CAD build for the part. Positions are in the model's coordinates, mm. A direction names the side the tool comes from. Coordinates: 2 decimals unless noted, no trailing zeros. Loops run counter-clockwise (first coordinate to the right, second up) from the corner with the lowest first, then second, coordinate; pieces in that order, holes last. Notation, with made-up numbers: M 1,37 L 52,37 A23 ccw 52,65 Z; hole C 27,-22 d11. An arc over 180 degrees is marked long. Answer as a JSON object with one key per item and string values. Group by question number.
```python
from build123d import *

# Parameters (mm, degrees)
F5_DEPTH = 4
F0_R     = 4.124509
F6_DEPTH = 32.004
F4_R     = 2.55
F7_DEPTH = 18.542
F2_R     = 2.55
F8_DEPTH = 16.764
F3_R     = 2.55
F9_DEPTH = 10.668


with BuildPart() as f5:
    # F1 (on Front) → F5 (new body)
    with BuildSketch(Plane.XZ):
        with BuildLine():
            ThreePointArc((-4.3, 101.097035), (-13.280256, 97.377291), (-17, 88.397035))
            Line((-17, 88.397035), (-17, 51.097035))
            Line((-17, 51.097035), (-64.3, 51.097035))
            ThreePointArc((-64.3, 51.097035), (-73.280256, 47.377291), (-77, 38.397035))
            Line((-77, 38.397035), (-77, -84.202965))
            ThreePointArc((-77, -84.202965), (-73.280256, -93.183221), (-64.3, -96.902965))
            Line((-64.3, -96.902965), (58.3, -96.902965))
            ThreePointArc((58.3, -96.902965), (67.280256, -93.183221), (71, -84.202965))
            Line((71, -84.202965), (71, 88.397035))
            ThreePointArc((71, 88.397035), (67.280256, 97.377291), (58.3, 101.097035))
            Line((58.3, 101.097035), (-4.3, 101.097035))
        make_face()
    extrude(amount=F5_DEPTH)

    # F0 (on Front) → F6 (cut)
    with BuildSketch(Plane.XZ):
        with Locations((-52.453019, -40.648032)):
            Circle(F0_R)
        with Locations((19.184319, -38.372811)):
            Circle(F0_R)
        with Locations((0, 84.097035)):
            Circle(F0_R)
    extrude(amount=F6_DEPTH, mode=Mode.SUBTRACT)

    # F4 (on Front) → F7 (cut)
    with BuildSketch(Plane.XZ):
        with Locations((-54, -73.902965)):
            Circle(F4_R)
        with Locations((24.5, -73.902965)):
            Circle(F4_R)
    extrude(amount=F7_DEPTH, mode=Mode.SUBTRACT)

    # F2 (on Front) → F8 (cut)
    with BuildSketch(Plane.XZ):
        with Locations((-53.5, 38.597035)):
            Circle(F2_R)
        with Locations((-53.5, -17.902965)):
            Circle(F2_R)
    extrude(amount=F8_DEPTH, mode=Mode.SUBTRACT)

    # F3 (on Front) → F9 (cut)
    with BuildSketch(Plane.XZ):
        with Locations((41, 66.097035)):
            Circle(F3_R)
        with Locations((47.5, -15.652965)):
            Circle(F3_R)
    extrude(amount=F9_DEPTH, mode=Mode.SUBTRACT)


solid = f5.part
```
Item 1: Slice it at D-D, the plane x = 0. Write the cut outline in (y, z).
Item 2: Slice it at C-C, the plane y = -1.6. Count the separate pieces of the cut face and the enclosed holes in it, then the cut area to 3 significant figures.
Item 3: Slice it at B-B, the plane x = -54. Write the cut outline in (y, z).
Item 4: Drill centre lines: L1, parallel to Z at x = -53.5, y = -1.15; L2, parallel to Z at x = 47, y = -1.8; L3, parallel to Z at x = -54, y = -2.5. Where is each one in solid material? Low to high. Write a range as from..to.
Item 5: Tool access for faces 1 (the flat face through (-17, -2, 70)), 2 (the flat face through (-4, -4, 3)): list every direction of +Z, -Z, +X, -X, +Y, -Y with a clear straight run to the whole face (end or side of a thin tool).
Item 6: Pin check, flat tips, straight feed: pin 1 (6.5 mm diameter, centred on x = 24.5, z = -73.9, fed in from -Y); pin 2 (4.5 mm diameter, centred on x = -53.5, z = -17.9, fed in from +Y); pin 3 (2 mm diameter, centred on x = -28.5, y = -3, fed in from +Z); pin 4 (1.2 mm diameter, centred on y = -2.5, z = 68.5, fed in from -X). Stop position of each tip, or through.
Item 7: Pull direction X, two halves, no side cores. Call faces 3 (the flat face through (-4, -2, -96.903)), 4 (the cylindrical face through (44.952, -1.972, -15.541)), 5 (the cylindrical face through (67.378, -1.972, 97.278)), 6 (the cylindrical face through (-73.38, -1.97, -93.08)): released by +X, released by -X, zero draft, split by the parting line, or undercut.
Item 8: Slice it at A-A, the plane x = 41. Write the cut outline in (y, z), then the cut area to 3 significant figures.
Computed:
{
 "1": {"outline": "M -4,-96.9 L 0,-96.9 L 0,79.97 L -4,79.97 Z; M -4,88.22 L 0,88.22 L 0,101.1 L -4,101.1 Z"},
 "2": {"separate pieces": "1", "enclosed holes": "9", "area": "25,800 mm2"},
 "3": {"outline": "M -4,-96.9 L 0,-96.9 L 0,-76.45 L -4,-76.45 Z; M -4,-71.35 L 0,-71.35 L 0,-44.47 L -4,-44.47 Z; M -4,-36.82 L 0,-36.82 L 0,-20.4 L -4,-20.4 Z; M -4,-15.4 L 0,-15.4 L 0,36.1 L -4,36.1 Z; M -4,41.1 L 0,41.1 L 0,51.1 L -4,51.1 Z"},
 "4": {"L1": "-96.9..-76.4, -71.4..-44.64, -36.66..-20.45, -15.35..36.05, 41.15..51.1", "L2": "-96.9..-18.15, -13.15..101.1", "L3": "-96.9..-76.45, -71.35..-44.47, -36.82..-20.4, -15.4..36.1, 41.1..51.1"},
 "5": {"face 1": "+Z, -X, +Y, -Y", "face 2": "+Z, -Z, +X, -X, -Y"},
 "6": {"pin 1": "y = -4", "pin 2": "through", "pin 3": "z = 51.1", "pin 4": "x = -17"},
 "7": {"face 3": "zero draft", "face 4": "undercut", "face 5": "released by +X", "face 6": "released by -X"},
 "8": {"outline": "M -4,-96.9 L 0,-96.9 L 0,63.55 L -4,63.55 Z; M -4,68.65 L 0,68.65 L 0,101.1 L -4,101.1 Z", "area": "772 mm2"}
}
